Could you check a few things on this model? Use its own coordinates, in mm. Face numbers are marked on the shaded views. A direction names the side the tool comes from. Round coordinates to 2 decimals unless told otherwise and drop trailing zeros. Write each loop counter-clockwise with the first axis right and the second up, starting at its lowest first coordinate (ties: lowest second). Pieces come first, ordered by that corner, then holes. Notation, with made-up numbers: (4.25, 1) - (36.25, 1) arc R22 cw to (36.25, 30) - close; hole circle Ø6 at (61.5, 54.25). An arc over 180 degrees is marked (long way). Write each question's results on one line, items separated by ' | '. Start each with the question number.
(1) Imagine slicing it at B-B on x = 0. Write out the boundary of the cut face in (y, z).
(2) For P1, Ø1.5, axis at x = -12.5, z = 7, coming from the +Y side; P2, Ø7, axis at x = -10.5, y = -24.5, coming from the +Z side; P3, Ø1, axis at x = -6, z = 0.5, coming from the -Y side, each with a flat end and sliding along its axis, tell me the tip position at first contact or that it passes through.
(3) Imagine slicing it at A-A on y = 0. Write out the boundary of the cut face in (x, z).
(4) On a 3-axis mill with a long thin cutter (end or side, diameter ignored), from which of +Z, -Z, +X, -X, +Y, -Y can I reach the whole of each face in a straight line? I mean the marked faces 1 and 2. Say none if no direction works.
(5) Thinking about a two-plate mould opening in X: for the marked faces 3, 4, 5 and 6, which applies, +X half, -X half, draft (parallel to the pull), parting line (faces both ways), or undercut?
(6) Imagine slicing it at C-C on y = -21. Write out the boundary of the cut face in (x, z).
(7) Imagine slicing it at D-D on z = 1.75. Write out the boundary of the cut face in (x, y), then the cut area to 3 significant figures.
(8) Please list where these lines run through material, in increasing order: line 1 (X direction, y = 0, z = -11.5); line 2 (Y direction, x = -18, z = -11.25); line 3 (Y direction, x = -13.5, z = 3.5). Write a range as [from, to].
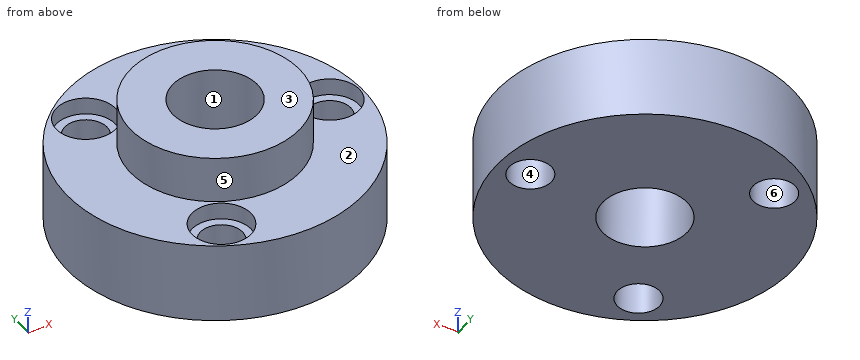
```python
from build123d import *

# Parameters (mm, degrees)
F0_R     = 20
F0_R_2   = 10
F1_DEPTH = 15
F2_R     = 35
F2_R_2   = 5
F2_R_3   = 10
F3_DEPTH = 15
F4_R     = 35
F4_R_2   = 7
F4_R_3   = 20
F5_DEPTH = 4


with BuildPart() as f1:
    # F0 (on Top) → F1 (new body)
    with BuildSketch(Plane.XY):
        Circle(F0_R)
        Circle(F0_R_2, mode=Mode.SUBTRACT)
    extrude(amount=F1_DEPTH)

    # F2 (on face) → F3 (join)
    with BuildSketch(Plane(origin=(0, 0, 0), x_dir=(1, 0, 0), z_dir=(0, 0, -1))):
        Circle(F2_R)
        with Locations((-17.977587, -20.810006)):
            Circle(F2_R_2, mode=Mode.SUBTRACT)
        with Locations((-13.474644, 23.972567)):
            Circle(F2_R_2, mode=Mode.SUBTRACT)
        Circle(F2_R_3, mode=Mode.SUBTRACT)
        with Locations((27.5, 0)):
            Circle(F2_R_2, mode=Mode.SUBTRACT)
    extrude(amount=F3_DEPTH)

    # F4 (on face) → F5 (join)
    with BuildSketch(Plane.XY):
        Circle(F4_R)
        with Locations((-13.474644, -23.972567)):
            Circle(F4_R_2, mode=Mode.SUBTRACT)
        with Locations((-17.977587, 20.810006)):
            Circle(F4_R_2, mode=Mode.SUBTRACT)
        Circle(F4_R_3, mode=Mode.SUBTRACT)
        with Locations((27.5, 0)):
            Circle(F4_R_2, mode=Mode.SUBTRACT)
    extrude(amount=F5_DEPTH)


solid = f1.part
```
Response:
1) outline: (-35, -15) - (-10, -15) - (-10, 15) - (-20, 15) - (-20, 4) - (-35, 4) - close; (10, -15) - (35, -15) - (35, 4) - (20, 4) - (20, 15) - (10, 15) - close
2) P1: y = 16.18 | P2: z = 0 | P3: y = -34.57
3) outline: (-35, -15) - (-10, -15) - (-10, 15) - (-20, 15) - (-20, 4) - (-35, 4) - close; (10, -15) - (22.5, -15) - (22.5, 0) - (20.5, 0) - (20.5, 4) - (20, 4) - (20, 15) - (10, 15) - close; (32.5, -15) - (35, -15) - (35, 4) - (34.5, 4) - (34.5, 0) - (32.5, 0) - close
4) face 1: +Z, -Z | face 2: +Z
5) face 3: draft | face 4: undercut | face 5: parting line | face 6: undercut
6) outline: (-28, -15) - (-17.5, -15) - (-17.5, 0) - (-19.81, 0) - (-19.81, 4) - (-28, 4) - close; (-9.45, -15) - (28, -15) - (28, 4) - (-7.14, 4) - (-7.14, 0) - (-9.45, 0) - close
7) outline: circle Ø70 at (0, 0); hole circle Ø14 at (-17.98, 20.81); hole circle Ø14 at (-13.47, -23.97); hole circle Ø20 at (0, 0); hole circle Ø14 at (27.5, 0) | area: 3,070 mm²
8) line 1: [-35, -10], [10, 22.5], [32.5, 35] | line 2: [-30.02, -26.1], [-21.85, 15.81], [25.81, 30.02] | line 3: [-32.29, -30.97], [-16.97, 15.43], [26.19, 32.29]
